Geometry: final body of the model. Coordinates: model frame, mm. Round coordinates to 2 decimals unless told otherwise and drop trailing zeros. Loops run counter-clockwise (first coordinate to the right, second up) from the corner with the lowest first, then second, coordinate; pieces in that order, holes last. Notation, with made-up numbers: M -23.75,-30 L -15.75,-30 A35 ccw -15.75,9 Z; hole C 74,-36 d8. An arc over 180 degrees is marked long. Answer as a JSON object with one key per item and string values.
from build123d import *

# Parameters (mm, degrees)
F0_W     = 60
F0_H     = 43
F0_R     = 6
F1_DEPTH = 34
F2_R     = 2.75
F3_DEPTH = 34.001
F4_R     = 2.75
F5_DEPTH = 43.001


with BuildPart() as f1:
    # F0 (on Front) → F1 (new body)
    with BuildSketch(Plane.XZ):
        Rectangle(F0_W, F0_H)
        with Locations((0, 3.5)):
            Circle(F0_R, mode=Mode.SUBTRACT)
    extrude(amount=-F1_DEPTH)

    # F2 (on face) → F3 (cut, through all)
    with BuildSketch(Plane.XZ):
        with Locations((23, 3.5)):
            Circle(F2_R)
        with Locations((-23, -14.5)):
            Circle(F2_R)
        with Locations((23, -14.5)):
            Circle(F2_R)
        with Locations((-23, 3.5)):
            Circle(F2_R)
    extrude(amount=-F3_DEPTH, mode=Mode.SUBTRACT)

    # F4 (on face) → F5 (cut, through all)
    with BuildSketch(Plane.XY.offset(21.5)):
        with Locations((-23, 19)):
            Circle(F4_R)
        with Locations((-23, 6)):
            Circle(F4_R)
        with Locations((23, 6)):
            Circle(F4_R)
        with Locations((23, 19)):
            Circle(F4_R)
    extrude(amount=-F5_DEPTH, mode=Mode.SUBTRACT)


solid = f1.part
1) Section query B-B (y = 10). Return the cut outline in (x, z), and give its area (3 significant figures).
Results:
{"outline": "M -30,-21.5 L 30,-21.5 L 30,21.5 L -30,21.5 Z; hole C -23,-14.5 d5.5; hole C -23,3.5 d5.5; hole C 0,3.5 d12; hole C 23,-14.5 d5.5; hole C 23,3.5 d5.5", "area": "2,370 mm2"}
2) Ray query, line 1 (Y direction, x = -23, z = -5.75); line 2 (Z direction, x = 23, y = 1.5); line 3 (X direction, y = 2.5, z = -14.5). Return the intervals inside material, ascending.
Results:
{"line 1": "0 to 3.25, 8.75 to 16.25, 21.75 to 34", "line 2": "-21.5 to -17.25, -11.75 to 0.75, 6.25 to 21.5", "line 3": "-30 to -25.75, -20.25 to 20.25, 25.75 to 30"}
3) Section query C-C (z = -1). Return the cut outline in (x, y), and give its area (3 significant figures).
Results:
{"outline": "M -30,0 L -3.97,0 L -3.97,34 L -30,34 Z; M 3.97,0 L 30,0 L 30,34 L 3.97,34 Z; hole C -23,6 d5.5; hole C -23,19 d5.5; hole C 23,6 d5.5; hole C 23,19 d5.5", "area": "1,680 mm2"}
4) Pin query (flat end, axial travel): P1, Ø3.5, axis at x = -23, y = 6, coming from the +Z side; P2, Ø7, axis at x = 23, z = 3.5, coming from the -Y side. Return the tip coordinate at first contact, or that it passes through.
Results:
{"P1": "through", "P2": "y = 0"}
5) Section query A-A (z = -9.5). Return the cut outline in (x, y), and give its area (3 significant figures).
Results:
{"outline": "M -30,0 L 30,0 L 30,34 L -30,34 Z; hole C -23,6 d5.5; hole C -23,19 d5.5; hole C 23,6 d5.5; hole C 23,19 d5.5", "area": "1,940 mm2"}
6) Section query D-D (x = -23). Count the separate pieces of the cut face and the enclosed holes in it, and give its area (3 significant figures).
Results:
{"separate pieces": "9", "enclosed holes": "0", "area": "736 mm2"}
7) Pull-direction query (Z, two-part tool) for faces 1 (the flat face through (0, 0, -4)), 2 (the cylindrical face through (-25.747, 12.409, -14.379)); classes: +Z half, -Z half, draft (parallel to the pull), parting line (faces both ways), or undercut.
Results:
{"face 1": "draft", "face 2": "undercut"}
